Geometry: final body of the model. Coordinates: model frame, mm. Face numbers are marked on the shaded views. Give positions to 0.01 mm unless a question says otherwise; leave off trailing zeros. Loops run counter-clockwise (first coordinate to the right, second up) from the corner with the lowest first, then second, coordinate; pieces in that order, holes last. Notation, with made-up numbers: (72, -26.75) - (115, -26.75) arc R27 cw to (115, 5.25) - close; hole circle Ø10 at (45, 82.25). An arc over 180 degrees is marked (long way). Answer in a Markdown table with one row per item.
from build123d import *

# Parameters (mm, degrees)
SKETCH3_R           = 31.75
BOSS_EXTRUDE1_DEPTH = 12.7
SKETCH4_R           = 22.225
CUT_EXTRUDE1_DEPTH  = 10.16
CUT_EXTRUDE2_DEPTH  = 10.16
SKETCH8_R           = 4.694761347
BOSS_EXTRUDE2_DEPTH = 16.51
SKETCH9_R           = 2.54
CUT_EXTRUDE3_DEPTH  = 10.16
SKETCH10_W          = 2.065443221
SKETCH10_H          = 12.7


with BuildPart() as part:
    # Sketch3 → Boss-Extrude1 (new body)
    with BuildSketch(Plane(origin=(0, 0, 0), x_dir=(1, 0, 0), z_dir=(0, 1, 0))):
        with Locations(Location((0, 0, 0), (0, 0, 270))):
            Circle(SKETCH3_R)
    extrude(amount=BOSS_EXTRUDE1_DEPTH)

    # Sketch4 → Cut-Extrude1 (cut)
    with BuildSketch(Plane(origin=(0, 12.7, 0), x_dir=(1, 0, 0), z_dir=(0, 1, 0))):
        with Locations(Location((0, 0, 0), (0, 0, 270))):
            Circle(SKETCH4_R)
    extrude(amount=-CUT_EXTRUDE1_DEPTH, mode=Mode.SUBTRACT)

    # Sketch7 → Cut-Extrude2 (cut)
    with BuildSketch(Plane(origin=(0, 2.54, 0), x_dir=(1, 0, 0), z_dir=(0, 1, 0))):
        with BuildLine():
            ThreePointArc((-15.229385619, -16.18692184), (-5.02164827, -21.65025805), (6.548839828, -21.238251385))
            add(Edge.make_bspline(
                [(-15.229385619, -16.18692184), (3.307519141, 7.259643736), (6.548839828, -21.238251385)],
                knots=[0, 0, 0, 1, 1, 1], degree=2))
        make_face()
        with BuildLine():
            ThreePointArc((13.050551616, -17.989822887), (19.536316665, -10.596365234), (22.196363392, -1.127863993))
            add(Edge.make_bspline(
                [(13.050551616, -17.989822887), (-5.30189954, 6.172036524), (22.196363392, -1.127863993)],
                knots=[0, 0, 0, 1, 1, 1], degree=2))
        make_face()
        with BuildLine():
            ThreePointArc((21.254913667, 6.494556954), (15.531294033, 15.897469316), (5.997580887, 21.400459072))
            add(Edge.make_bspline(
                [(5.997580887, 21.400459072), (-2.424740226, -1.907285391), (21.254913667, 6.494556954)],
                knots=[0, 0, 0, 1, 1, 1], degree=2))
        make_face()
        with BuildLine():
            ThreePointArc((0, 22.225), (-11.007401994, 19.307711577), (-19.125106224, 11.321702033))
            add(Edge.make_bspline(
                [(0, 22.225), (0.733559441, -2.419288654), (-19.125106224, 11.321702033)],
                knots=[0, 0, 0, 1, 1, 1], degree=2))
        make_face()
        with BuildLine():
            ThreePointArc((-21.0799969, 7.041615986), (-22.014836277, -3.049198044), (-18.372518541, -12.506046036))
            add(Edge.make_bspline(
                [(-21.0799969, 7.041615986), (6.067470104, 0.607937187), (-18.372518541, -12.506046036)],
                knots=[0, 0, 0, 1, 1, 1], degree=2))
        make_face()
    extrude(amount=-CUT_EXTRUDE2_DEPTH, mode=Mode.SUBTRACT)

    # Sketch8 → Boss-Extrude2 (add)
    with BuildSketch(Plane(origin=(0, 2.54, 0), x_dir=(1, 0, 0), z_dir=(0, 1, 0))):
        with Locations(Location((0, 0, 0), (0, 0, 270))):
            Circle(SKETCH8_R)
    extrude(amount=BOSS_EXTRUDE2_DEPTH)

    # Sketch9 → Cut-Extrude3 (cut)
    with BuildSketch(Plane(origin=(0, 19.05, 0), x_dir=(1, 0, 0), z_dir=(0, 1, 0))):
        with Locations(Location((0, 0, 0), (0, 0, 270))):
            Circle(SKETCH9_R)
    extrude(amount=-CUT_EXTRUDE3_DEPTH, mode=Mode.SUBTRACT)

    # Sketch10 → Revolve1 (revolve)
    with BuildSketch(Plane.XY, mode=Mode.PRIVATE) as revolve1_sk:
        with Locations((-32.782721611, 6.35)):
            Rectangle(SKETCH10_W, SKETCH10_H)
    revolve(revolve1_sk.sketch.rotate(Axis((0, 24.137894977, 0), (0, -1, 0)), 270), axis=Axis((0, 24.137894977, 0), (0, -1, 0)))


solid = part.part
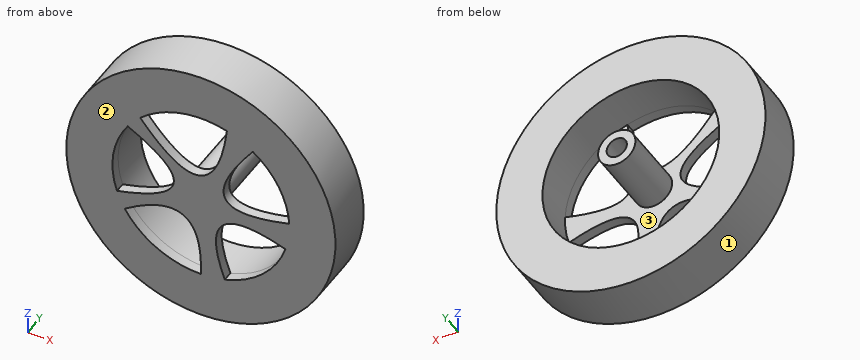
Q1. Material intervals for line 1 along X through (y, z) = (9.5, 0) (3 decimals); line 2 along X through (y, z) = (8, 0) (3 decimals); line 3 along X through (y, z) = (1, 7), sorted ascending.
Check values:
| item | result |
|---|---|
| line 1 | -33.815 to -22.225, -4.695 to -2.54, 2.54 to 4.695, 22.225 to 33.815 |
| line 2 | -33.815 to -22.225, -4.695 to 4.695, 22.225 to 33.815 |
| line 3 | -33.08 to -21.09, -10.05 to -5.84, 1.79 to 6.39, 21.09 to 33.08 |
Q2. First-contact query: pin 1 (3 mm diameter, centred on x = -5.5, z = -1, fed in from +Y); pin 2 (3 mm diameter, centred on y = 2.5, z = 7, fed in from -X); pin 3 (3 mm diameter, centred on y = 16.5, z = -2.5, fed in from -X); pin 4 (4 mm diameter, centred on x = -3, z = 26.5, fed in from +Y). Flat tips, straight axial feed; report the tip coordinate or a pass-through.
Check values:
| item | result |
|---|---|
| pin 1 | y = 19.05 |
| pin 2 | x = -33.37 |
| pin 3 | x = -4.59 |
| pin 4 | y = 12.7 |
Q3. Cut plane C-C (z = -10). Give the number of separate pieces and of enclosed holes in the cut face, and give its area (3 significant figures).
Check values:
| item | result |
|---|---|
| separate pieces | 3 |
| enclosed holes | 0 |
| area | 338 mm² |
Q4. Cut plane B-B (y = 14). Output: boundary loops of the cut face in (x, z), and give its area (3 significant figures).
Check values:
| item | result |
|---|---|
| outline | circle Ø9.39 at (0, 0); hole circle Ø5.08 at (0, 0) |
| area | 49.0 mm² |
Q5. Draft query along X for the marked faces 1, 2 and 3. Return one class per face: pulls with the +X half, pulls with the -X half, needs draft (parallel to the pull), parting line crosses it, or undercut.
Check values:
| item | result |
|---|---|
| face 1 | parting line crosses it |
| face 2 | needs draft |
| face 3 | undercut |
Q6. Cut plane A-A (y = 10.25). Output: boundary loops of the cut face in (x, z) (3 decimals), and give its area (3 significant figures).
Check values:
| item | result |
|---|---|
| outline | circle Ø67.631 at (0, 0); circle Ø9.39 at (0, 0); hole circle Ø44.45 at (0, 0); hole circle Ø5.08 at (0, 0) |
| area | 2,090 mm² |
